```python
from build123d import *
from OCP.BRepFilletAPI import BRepFilletAPI_MakeChamfer

# Parameters (mm, degrees)
BOSS_EXTRUDE1_DEPTH = 0.4
BOSS_EXTRUDE2_DEPTH = 6
CHAMFER1_SIZE       = 6.4
CHAMFER1_SIZE_2     = 3.955417619
BOSS_EXTRUDE3_DEPTH = 1
CUT_EXTRUDE1_DEPTH  = 1.075
CIRPATTERN1_COUNT   = 5
CHAMFER2_SIZE       = 0.2
CHAMFER2_SIZE2      = 0.546410162
CUT_EXTRUDE2_REACH  = 96.106
SKETCH9_R           = 20
FILLET1_R           = 2
CHAMFER3_SIZE       = 0.5
BOSS_EXTRUDE6_DEPTH = 6
CIRPATTERN4_COUNT   = 5


with BuildPart() as part:
    # Sketch1 → Boss-Extrude1 (new body)
    with BuildSketch(Plane(origin=(0, 0, 0), x_dir=(1, 0, 0), z_dir=(0, 1, 0))):
        Polygon((0, 68.052064668), (-64.72135955, 21.029244485), (-40, -55.055276819), (40, -55.055276819), (64.72135955, 21.029244485), align=None)
    extrude(amount=BOSS_EXTRUDE1_DEPTH)

    # Sketch2 → Boss-Extrude2 (add)
    with BuildSketch(Plane(origin=(0, 0.4, 0), x_dir=(1, 0, 0), z_dir=(0, 1, 0))):
        Polygon((64.72135955, 21.029244485), (0, 68.052064668), (-64.72135955, 21.029244485), (-40, -55.055276819), (40, -55.055276819), align=None)
        Polygon((57.667936522, 18.737448417), (0, 60.635656803), (-57.667936522, 18.737448417), (-35.640744832, -49.055276819), (35.640744832, -49.055276819), align=None, mode=Mode.SUBTRACT)
    extrude(amount=BOSS_EXTRUDE2_DEPTH)

    # Chamfer1
    # the kernel refuses this chamfer: 6.4, 3.955417619 mm, written as the material it takes off along each edge
    with BuildSketch(Plane(origin=(13.387481819, 6.4, -77.778639553), x_dir=(-0.011951463674796303, -0.9997932622810094, -0.0164497785251576), z_dir=(-0.8090169943749475, 0, 0.5877852522924732)), Plane(origin=(34.886436969, 6.4, 70.793205576), x_dir=(0.019337874441129724, -0.9997932622810094, 0.006283256289201955), z_dir=(0.30901699437494756, 0, -0.9510565162951536)), Plane(origin=(-56.547837576, 6.4, 55.055276819), x_dir=(0, -0.9997932622810094, 0.020333044471910092), z_dir=(1, 0, 0)), Plane(origin=(-69.834922581, 6.4, -36.767173242), x_dir=(-0.019337874441129724, -0.9997932622810094, 0.006283256289201957), z_dir=(0.3090169943749477, 0, 0.9510565162951535))) as chamfer1_piece_1:
        Polygon((CHAMFER1_SIZE * 0.999793262281, CHAMFER1_SIZE * 0.0203330444719), (-CHAMFER1_SIZE_2 * 0.0203330444711, CHAMFER1_SIZE_2 * 0.999793262243), (0, 0), align=None)
    extrude(amount=113.095675152, mode=Mode.SUBTRACT)
    with BuildSketch(Plane(origin=(78.108841369, 6.4, -11.3026696), x_dir=(-0.586953868721804, 0.05316829695991145, 0.8078726930593024), z_dir=(-0.8090169943749477, 0, -0.5877852522924728))) as chamfer1_piece_2:
        Polygon((CHAMFER1_SIZE_2 * 0.998585565749, -CHAMFER1_SIZE_2 * 0.0531682969579), (-CHAMFER1_SIZE * 0.0531682969599, -CHAMFER1_SIZE * 0.998585565787), (0, 0), align=None)
    extrude(amount=113.095675152, mode=Mode.SUBTRACT)

    # Sketch3 → Boss-Extrude3 (add, symmetric)
    with BuildSketch(Plane(origin=(20, 0, 0), x_dir=(0, 0, -1), z_dir=(1, 0, 0))):
        with BuildLine():
            Line((-54.842648148, 4.495096909), (-53.648646953, 2.275974881))
            Line((-53.648646953, 2.275974881), (-51.413238488, 5.892941672))
            Line((-51.413238488, 5.892941672), (-53.932055136, 5.968467319))
            ThreePointArc((-53.932055136, 5.968467319), (-54.812677044, 5.494647674), (-54.842648148, 4.495096909))
        make_face()
    boss_extrude3 = extrude(amount=BOSS_EXTRUDE3_DEPTH, both=True)

    # Sketch5 → Revolve1 (revolve)
    with BuildSketch(Plane(origin=(0, 4.968916553, 0), x_dir=(-1, 0, 0), z_dir=(0, 1, 0))):
        with BuildLine():
            Line((-21, 54.962026241), (-21, 53.962026241))
            Line((-21, 53.962026241), (-21.25, 53.962026241))
            ThreePointArc((-21.25, 53.962026241), (-21.186552813, 54.477414444), (-21, 54.962026241))
        make_face()
    revolve1 = revolve(axis=Axis((21, 4.968916553, 53.962026241), (1, 0, 0)))

    # Mirror1: Revolve1 across plane
    add(revolve1.mirror(Plane(origin=(20, 0, 0), x_dir=(0, 0, 1), z_dir=(1, 0, 0))))

    # Sketch6 → Cut-Extrude1 (cut, symmetric)
    with BuildSketch(Plane(origin=(-20, 0, 0), x_dir=(0, 0, -1), z_dir=(1, 0, 0))):
        with BuildLine():
            Line((-51.401250046, 6.292761979), (-50.043112911, 3.768583574))
            ThreePointArc((-50.043112911, 3.768583574), (-50.079078236, 2.569122655), (-51.135824526, 2.000539081))
            Line((-51.135824526, 2.000539081), (-54.000895716, 2.086447023))
            Line((-54.000895716, 2.086447023), (-51.401250046, 6.292761979))
        make_face()
    cut_extrude1 = extrude(amount=CUT_EXTRUDE1_DEPTH, both=True, mode=Mode.SUBTRACT)

    # Sketch8 → Cut-Revolve1 (revolve, cut)
    with BuildSketch(Plane(origin=(0, 3.2, 0), x_dir=(1, 0, 0), z_dir=(0, 1, 0))):
        with BuildLine():
            Line((-21.075, -51.0998592), (-21.475, -51.0998592))
            ThreePointArc((-21.475, -51.0998592), (-21.372366596, -50.467403668), (-21.075, -49.8998592))
            Line((-21.075, -49.8998592), (-21.075, -51.0998592))
        make_face()
    cut_revolve1 = revolve(axis=Axis((-21.075, 3.2, 51.0998592), (-1, 0, 0)), mode=Mode.SUBTRACT)

    # Mirror2: Cut-Revolve1 across plane
    add(cut_revolve1.mirror(Plane(origin=(-20, 0, 0), x_dir=(0, 0, 1), z_dir=(1, 0, 0))), mode=Mode.SUBTRACT)

    # CirPattern1: Boss-Extrude3, Revolve1, Cut-Extrude1, Cut-Revolve1 ×5 about axis
    cirpattern1_axis = Axis((0, 0, 0), (0, 1, 0))
    add([boss_extrude3.rotate(cirpattern1_axis, i * 360 / CIRPATTERN1_COUNT) for i in range(1, CIRPATTERN1_COUNT)])
    add([revolve1.rotate(cirpattern1_axis, i * 360 / CIRPATTERN1_COUNT) for i in range(1, CIRPATTERN1_COUNT)])
    add([cut_extrude1.rotate(cirpattern1_axis, i * 360 / CIRPATTERN1_COUNT) for i in range(1, CIRPATTERN1_COUNT)], mode=Mode.SUBTRACT)
    add([cut_revolve1.rotate(cirpattern1_axis, i * 360 / CIRPATTERN1_COUNT) for i in range(1, CIRPATTERN1_COUNT)], mode=Mode.SUBTRACT)

    # CirPattern1 copy 1 sketch → CirPattern1 copy 1 (revolve)
    with BuildSketch(Plane(origin=(12.360679775, 4.968916553, -38.042260652), x_dir=(0.30901699437494745, 0, -0.9510565162951535), z_dir=(0, 1, 0))):
        with BuildLine():
            Line((-21, -54.962026241), (-21, -53.962026241))
            Line((-21, -53.962026241), (-21.25, -53.962026241))
            ThreePointArc((-21.25, -53.962026241), (-21.186552813, -54.477414444), (-21, -54.962026241))
        make_face()
    revolve(axis=Axis((57.192259582, 4.968916553, -1.39489065), (0.30901699437494745, 0, -0.9510565162951535)))

    # CirPattern1 copy 2 sketch → CirPattern1 copy 2 (revolve)
    with BuildSketch(Plane(origin=(-32.360679775, 4.968916553, -23.511410092), x_dir=(-0.8090169943749473, 0, -0.5877852522924732), z_dir=(0, 1, 0))):
        with BuildLine():
            Line((-21, -54.962026241), (-21, -53.962026241))
            Line((-21, -53.962026241), (-21.25, -53.962026241))
            ThreePointArc((-21.25, -53.962026241), (-21.186552813, -54.477414444), (-21, -54.962026241))
        make_face()
    revolve(axis=Axis((16.346760315, 4.968916553, -54.824116073), (-0.8090169943749473, 0, -0.5877852522924732)))

    # CirPattern1 copy 3 sketch → CirPattern1 copy 3 (revolve)
    with BuildSketch(Plane(origin=(-32.360679775, 4.968916553, 23.511410092), x_dir=(-0.8090169943749476, 0, 0.587785252292473), z_dir=(0, 1, 0))):
        with BuildLine():
            Line((-21, -54.962026241), (-21, -53.962026241))
            Line((-21, -53.962026241), (-21.25, -53.962026241))
            ThreePointArc((-21.25, -53.962026241), (-21.186552813, -54.477414444), (-21, -54.962026241))
        make_face()
    revolve(axis=Axis((-47.089406101, 4.968916553, -32.488276486), (-0.8090169943749476, 0, 0.587785252292473)))

    # CirPattern1 copy 4 sketch → CirPattern1 copy 4 (revolve)
    with BuildSketch(Plane(origin=(12.360679775, 4.968916553, 38.042260652), x_dir=(0.30901699437494723, 0, 0.9510565162951536), z_dir=(0, 1, 0))):
        with BuildLine():
            Line((-21, -54.962026241), (-21, -53.962026241))
            Line((-21, -53.962026241), (-21.25, -53.962026241))
            ThreePointArc((-21.25, -53.962026241), (-21.186552813, -54.477414444), (-21, -54.962026241))
        make_face()
    revolve(axis=Axis((-45.449613795, 4.968916553, 34.745256969), (0.30901699437494723, 0, 0.9510565162951536)))

    # CirPattern1 copy 5 sketch → CirPattern1 copy 5 (revolve, cut)
    with BuildSketch(Plane(origin=(-12.360679775, 3.2, 38.042260652), x_dir=(-0.30901699437494745, 0, 0.9510565162951535), z_dir=(0, 1, 0))):
        with BuildLine():
            Line((-21.075, 51.0998592), (-21.475, 51.0998592))
            ThreePointArc((-21.475, 51.0998592), (-21.372366596, 50.467403668), (-21.075, 49.8998592))
            Line((-21.075, 49.8998592), (-21.075, 51.0998592))
        make_face()
    revolve(axis=Axis((42.750707455, 3.2, 33.789469474), (-0.30901699437494745, 0, 0.9510565162951535)), mode=Mode.SUBTRACT)

    # CirPattern1 copy 6 sketch → CirPattern1 copy 6 (revolve, cut)
    with BuildSketch(Plane(origin=(32.360679775, 3.2, 23.511410092), x_dir=(0.8090169943749473, 0, 0.5877852522924732), z_dir=(0, 1, 0))):
        with BuildLine():
            Line((-21.075, 51.0998592), (-21.475, 51.0998592))
            ThreePointArc((-21.475, 51.0998592), (-21.372366596, 50.467403668), (-21.075, 49.8998592))
            Line((-21.075, 49.8998592), (-21.075, 51.0998592))
        make_face()
    revolve(axis=Axis((45.346390251, 3.2, -30.216818603), (0.8090169943749473, 0, 0.5877852522924732)), mode=Mode.SUBTRACT)

    # CirPattern1 copy 7 sketch → CirPattern1 copy 7 (revolve, cut)
    with BuildSketch(Plane(origin=(32.360679775, 3.2, -23.511410092), x_dir=(0.8090169943749476, 0, -0.587785252292473), z_dir=(0, 1, 0))):
        with BuildLine():
            Line((-21.075, 51.0998592), (-21.475, 51.0998592))
            ThreePointArc((-21.475, 51.0998592), (-21.372366596, 50.467403668), (-21.075, 49.8998592))
            Line((-21.075, 49.8998592), (-21.075, 51.0998592))
        make_face()
    revolve(axis=Axis((-14.725097013, 3.2, -52.464490403), (0.8090169943749476, 0, -0.587785252292473)), mode=Mode.SUBTRACT)

    # CirPattern1 copy 8 sketch → CirPattern1 copy 8 (revolve, cut)
    with BuildSketch(Plane(origin=(-12.360679775, 3.2, -38.042260652), x_dir=(-0.30901699437494723, 0, -0.9510565162951536), z_dir=(0, 1, 0))):
        with BuildLine():
            Line((-21.075, 51.0998592), (-21.475, 51.0998592))
            ThreePointArc((-21.475, 51.0998592), (-21.372366596, 50.467403668), (-21.075, 49.8998592))
            Line((-21.075, 49.8998592), (-21.075, 51.0998592))
        make_face()
    revolve(axis=Axis((-54.447000692, 3.2, -2.208019668), (-0.30901699437494723, 0, -0.9510565162951536)), mode=Mode.SUBTRACT)

    # Chamfer2: one chamfer whose edges measure the first distance from different faces: ONE call of the kernel's chamfer builder (chamfer() names one face for all edges)
    chamfer2_edges_1 = [part.edges().sort_by_distance(p)[0] for p in [
        (-18.925, 4.084458277, 52.53094272),
        (-21.075, 4.084458277, 52.53094272),
    ]]
    chamfer2_edges_2 = [part.edges().sort_by_distance(p)[0] for p in [
        (-20, 2.079525493, 53.770059354),
        (-20, 6.08939106, 51.291826086),
    ]]
    chamfer2_side_2 = [part.faces().sort_by_distance(p)[0] for p in [
        (0.058075129, 3.129583761, 53.121087639),
    ]]
    chamfer2 = BRepFilletAPI_MakeChamfer(part.part.solid().wrapped)
    for e in chamfer2_edges_1:
        chamfer2.Add(CHAMFER2_SIZE, e.wrapped)
    for e in chamfer2_edges_2:
        chamfer2.Add(CHAMFER2_SIZE, CHAMFER2_SIZE2, e.wrapped, chamfer2_side_2[0].wrapped)  # the first distance lies on this face
    add(Compound.cast(chamfer2.Shape()), mode=Mode.REPLACE)

    # Sketch9 → Cut-Extrude2 (cut, up to next)
    with BuildSketch(Plane(origin=(0, 0.4, 0), x_dir=(1, 0, 0), z_dir=(0, 1, 0)), mode=Mode.PRIVATE) as cut_extrude2_sk1:
        with Locations(Location((0, 0, 0), (0, 0, 270))):
            Circle(SKETCH9_R)
    cut_extrude2_tool1 = extrude(cut_extrude2_sk1.sketch, amount=-CUT_EXTRUDE2_REACH, mode=Mode.PRIVATE) & part.part
    add(cut_extrude2_tool1.solids().sort_by_distance((0, 0.4, 0))[0], mode=Mode.SUBTRACT)

    # Sketch13 → Revolve2 (revolve)
    with BuildSketch(Plane(origin=(0, 0, 0), x_dir=(0, 0, -1), z_dir=(1, 0, 0)), mode=Mode.PRIVATE) as revolve2_sk:
        Polygon((-16.5, 0), (-16.5, 30), (-13.9, 30), (-13.9, 31.8), (-20, 31.8), (-20, 0), align=None)
    revolve(revolve2_sk.sketch.rotate(Axis((0, 0, 0), (0, 1, 0)), 180), axis=Axis((0, 0, 0), (0, 1, 0)))

    # Fillet1
    fillet1_edges = [part.edges().sort_by_distance(p)[0] for p in [
        (0, 31.8, 20),
    ]]
    fillet(fillet1_edges, radius=FILLET1_R)

    # Chamfer3
    chamfer3_edges = [part.edges().sort_by_distance(p)[0] for p in [
        (0, 30, 13.9),
        (0, 31.8, 13.9),
    ]]
    chamfer(chamfer3_edges, length=CHAMFER3_SIZE)

    # Sketch14 → Boss-Extrude6 (add)
    with BuildSketch(Plane(origin=(0, 0.4, 0), x_dir=(1, 0, 0), z_dir=(0, 1, 0))):
        with BuildLine():
            Line((-10.078744846, 17.274805421), (-27.215934272, 40.862123115))
            Line((-27.215934272, 40.862123115), (-30.45200225, 38.510982106))
            Line((-30.45200225, 38.510982106), (-13.314812824, 14.923664412))
            ThreePointArc((-13.314812824, 14.923664412), (-11.755705046, 16.180339887), (-10.078744846, 17.274805421))
        make_face()
    boss_extrude6 = extrude(amount=BOSS_EXTRUDE6_DEPTH)

    # CirPattern4: Boss-Extrude6 ×5 about axis
    cirpattern4_axis = Axis((0, 0, 0), (0, 1, 0))
    for i in range(1, CIRPATTERN4_COUNT):
        add(boss_extrude6.rotate(cirpattern4_axis, i * 360 / CIRPATTERN4_COUNT))


solid = part.part
```
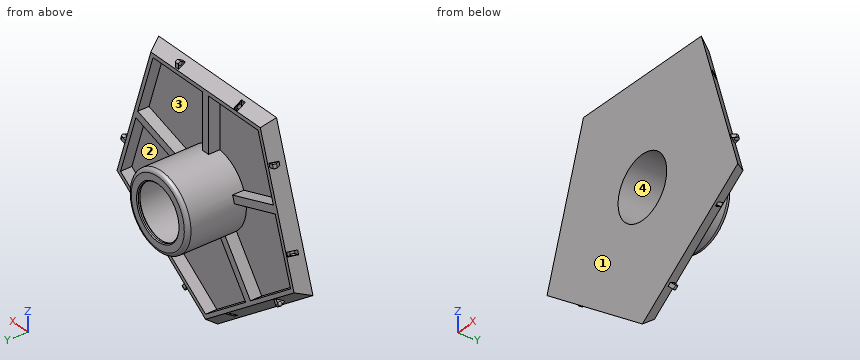
The model under review builds one solid part; all positions refer to its coordinate system, in mm. Face numbers are marked on the shaded views. A direction names the side the tool comes from. Give positions to 0.01 mm unless a question says otherwise; leave off trailing zeros. Write each loop counter-clockwise with the first axis right and the second up, starting at its lowest first coordinate (ties: lowest second). Pieces come first, ordered by that corner, then holes. Notation, with made-up numbers: M 2,20 L 17,20 A13 ccw 17,26 Z; hole C 11,0 d1. An arc over 180 degrees is marked long. Write each question's results on one line, items separated by ' | '. Start each with the question number.
1. Mouldability with a two-part tool opening along Z and no side actions: class the marked faces 1 and 2 as released by +Z, released by -Z, zero draft, split by the parting line, or undercut.
2. We need section A-A (y = 21). Write out the cut boundary in (x, z).
3. We need section B-B (z = 21.5). Write out the cut boundary in (x, y), and give its area (3 significant figures).
4. For probe 1 along X at (y, z) = (31.05, 0); probe 2 along Y at (x, z) = (-23, -41.5); probe 3 along X at (y, z) = (13.5, 0), list the stretches that pass through material, from the lowest coordinate up. Write a range as [from, to].
5. Insertion check: pin 1 Ø10 at (x, z) = (-8, -47.5) entering from +Y; pin 2 Ø3 at (x, y) = (-25.5, 4) entering from -Z; pin 3 Ø1.8 at (x, y) = (25, 3.5) entering from -Z. Each pin has a flat end and moves straight along its axis. Give the tip position at first contact, or say it passes through.
6. For the marked faces 3 and 4, list the 3-axis set-ups (+Z, -Z, +X, -X, +Y, -Y) from which the entire face can be reached by the end or side of a thin tool; tool diameter is ignored.
7. We need section C-C (z = 38.5). Write out the cut boundary in (x, y).
Results found:
1) face 1: zero draft | face 2: undercut
2) outline: C 0,0 d40; hole C 0,0 d33
3) outline: M -50.9,0 L 50.9,0 L 46.74,6.4 L 44.59,6.4 L 44.59,0.4 L 2,0.4 L 2,6.4 L -2,6.4 L -2,0.4 L -44.59,0.4 L -44.59,6.4 L -46.74,6.4 Z | area: 114 mm^2
4) probe 1: x = [-19.56, -13.9], [13.9, 19.56] | probe 2: y = [0, 0.4] | probe 3: x = [-20, -16.5], [16.5, 20]
5) pin 1: stops at y = 0.4 | pin 2: stops at z = -48.05 | pin 3: stops at z = -48.16
6) face 3: +Y | face 4: -Y
7) outline: M -45.38,0 L 45.38,0 L 41.22,6.4 L 39.07,6.4 L 39.07,0.4 L 2,0.4 L 2,6.4 L -2,6.4 L -2,0.4 L -39.07,0.4 L -39.07,6.4 L -41.22,6.4 Z
